Can you work these out from the model? Positions are in its coordinate system, mm. A direction names the side the tool comes from. Round coordinates to 2 decimals unless told otherwise and drop trailing zeros. Loops run counter-clockwise (first coordinate to the right, second up) from the corner with the lowest first, then second, coordinate; pieces in that order, holes last. Notation, with made-up numbers: (0.25, 68) -> (43.25, 68) arc R20 ccw to (43.25, 105) -> close; hole circle Ø9 at (37.5, -1.5). An arc over 180 degrees is marked (long way). Use a Markdown table: item, result.
from build123d import *

# Parameters (mm, degrees)
F0_W     = 508
F0_H     = 300
F1_DEPTH = 21


with BuildPart() as f1:
    # F0 (on Front) → F1 (new body)
    with BuildSketch(Plane.XZ):
        with Locations((254, 150)):
            Rectangle(F0_W, F0_H)
        with BuildLine():
            ThreePointArc((64.245627, 208.035878), (254, 250), (443.754373, 208.035878))
            ThreePointArc((443.754373, 208.035878), (456.616189, 193.840292), (455.418317, 174.722078))
            ThreePointArc((455.418317, 174.722078), (254, 50), (52.581683, 174.722078))
            ThreePointArc((52.581683, 174.722078), (51.383811, 193.840292), (64.245627, 208.035878))
        make_face(mode=Mode.SUBTRACT)
    extrude(amount=F1_DEPTH)


solid = f1.part
1. I want a section at A-A (y = -6.5). Please give me the cut outline in (x, z), plus the area to 3 significant figures.
Answer sheet:
| item | result |
|---|---|
| outline | (0, 0) -> (508, 0) -> (508, 300) -> (0, 300) -> close; hole (52.58, 174.72) arc R225 ccw to (455.42, 174.72) arc R24.63 ccw to (443.75, 208.04) arc R450 ccw to (64.25, 208.04) arc R24.63 ccw to start |
| area | 92,300 mm² |
2. I want a section at B-B (z = 108.5). Please give me the cut outline in (x, y), plus the area to 3 significant figures.
Answer sheet:
| item | result |
|---|---|
| outline | (0, -21) -> (102.66, -21) -> (102.66, 0) -> (0, 0) -> close; (405.34, -21) -> (508, -21) -> (508, 0) -> (405.34, 0) -> close |
| area | 4,310 mm² |
3. I need wall thicknesses on line 1 (X direction, y = -7.25, z = 154); line 2 (X direction, y = -8, z = 95.5); line 3 (Z direction, x = 163, y = -7.5). Which ranges of each line are inside material? Lowest first, please.
Answer sheet:
| item | result |
|---|---|
| line 1 | x = 0 to 64.31, 443.69 to 508 |
| line 2 | x = 0 to 118.34, 389.66 to 508 |
| line 3 | z = 0 to 69.22, 240.7 to 300 |
4. If we mould it in two halves opening along Z, with no side actions, what happens to faces 3 (the flat face through (0, -10, 148)), 4 (the flat face through (250, -10, 300)), 5 (the cylindrical face through (456.524, -10.353, 194.1))? For each: +Z half, -Z half, draft (parallel to the pull), parting line (faces both ways), or undercut.
Answer sheet:
| item | result |
|---|---|
| face 3 | draft |
| face 4 | +Z half |
| face 5 | undercut |
5. I want a section at C-C (x = 279.5). Please give me the cut outline in (y, z), plus the area to 3 significant figures.
Answer sheet:
| item | result |
|---|---|
| outline | (-21, 0) -> (0, 0) -> (0, 51.45) -> (-21, 51.45) -> close; (-21, 249.28) -> (0, 249.28) -> (0, 300) -> (-21, 300) -> close |
| area | 2,150 mm² |
6. Which directions (+Z, -Z, +X, -X, +Y, -Y) give clear straight access to the entire face, cutting with the end or side of a thin tool? Please do faces 1 (the flat face through (250, 0, 252)), 2 (the cylindrical face through (251.26, -10.35, 249.99)).
Answer sheet:
| item | result |
|---|---|
| face 1 | +Z, -Z, +X, -X, +Y |
| face 2 | +Y, -Y |
